Here's the drawing with two shaded views (mm, measured from the low corner). I have some questions. A direction names the side the tool comes from. Round coordinates to 2 decimals unless told otherwise and drop trailing zeros. Order: outer loops, then holes, each group sorted by start corner. A loop starts at its lowest first (then second) coordinate and runs counter-clockwise, first axis right, second up. Notation, with made-up numbers: (-15.5, 62.25) -> (23.5, 62.25) arc R26 ccw to (23.5, 86.25) -> close; hole circle Ø7 at (1, 39.5). An arc over 180 degrees is marked (long way). Use a Markdown table: item, result. Add a question column.
Q1. I need wall thicknesses on line 1 along Y through (x, z) = (3.1, 3.85); line 2 along Y through (x, z) = (0.5, 4); line 3 along X through (y, z) = (12.15, 4.05). Which ranges of each line are inside material? Lowest first, please. Write a range as [from, to].
Q2. For the marked faces 1 and 2, which set-ups out of +Z, -Z, +X, -X, +Y, -Y let a thin tool reach every point of the face, with its end or its side?
Q3. We'd pull the mould along X, two halves only. Please class the marked faces 3, 4 and 5: +X half, -X half, draft (parallel to the pull), parting line (faces both ways), or undercut.
Q4. If we section it at A-A on x = 3.1: List the corners of the cut face in (y, z) for me.
Q5. If we section it at C-C on y = 9.25: List the corners of the cut face in (x, z) for me, plus the area to 3 significant figures.
Q6. If we section it at D-D on x = 4.75: List the corners of the cut face in (y, z) for me.
Q7. If we section it at B-B on z = 3.1: List the corners of the cut face in (x, y) for me.
Q8. I'm going to push flat-ended pins straight in: pin 1 Ø1 at (x, z) = (2.5, 5.5) entering from -Y; pin 2 Ø2 at (x, y) = (3, 4.5) entering from -Z. Where does each tip first touch, or does it pass through?
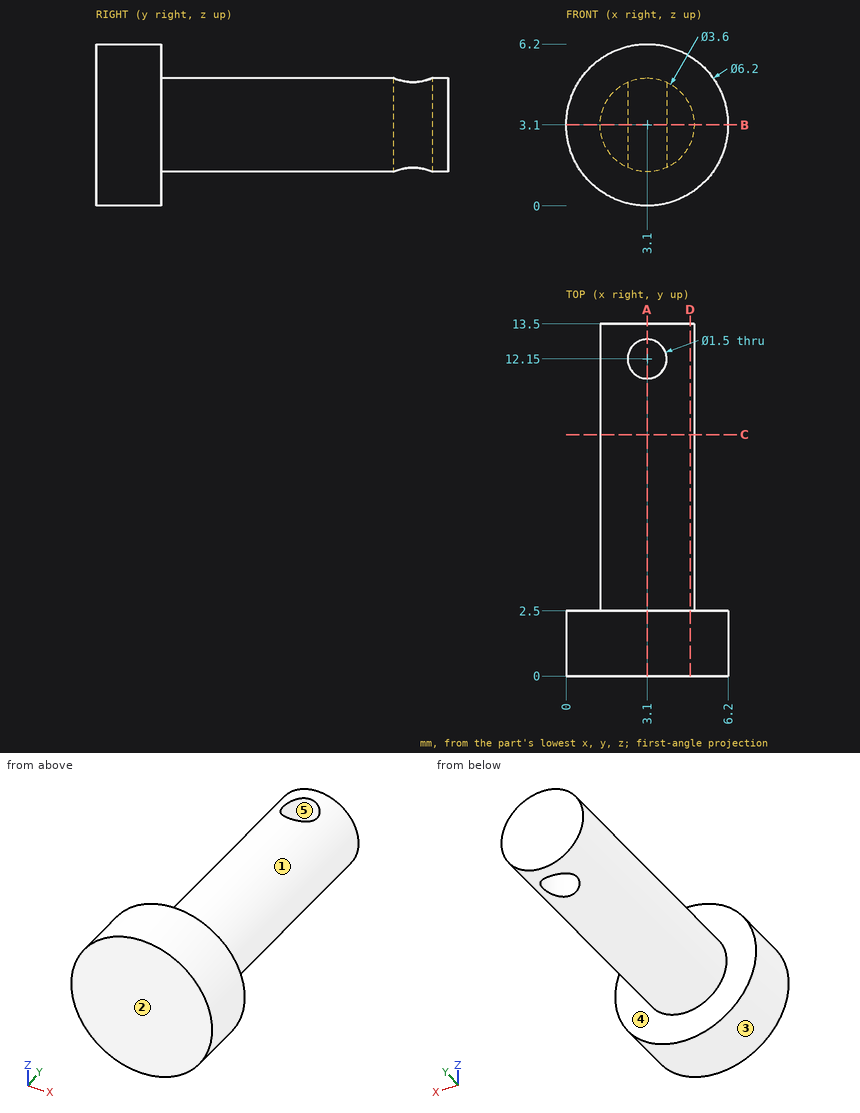
Answer below:
| question | item | result |
|---|---|---|
| 1 | line 1 | [0, 11.4], [12.9, 13.5] |
| 1 | line 2 | [0, 2.5] |
| 1 | line 3 | [1.57, 2.35], [3.85, 4.63] |
| 2 | face 1 | +Y |
| 2 | face 2 | +Z, -Z, +X, -X, -Y |
| 3 | face 3 | parting line |
| 3 | face 4 | draft |
| 3 | face 5 | undercut |
| 4 | outline | (0, 0) -> (2.5, 0) -> (2.5, 1.3) -> (11.4, 1.3) -> (11.4, 4.9) -> (2.5, 4.9) -> (2.5, 6.2) -> (0, 6.2) -> close; (12.9, 1.3) -> (13.5, 1.3) -> (13.5, 4.9) -> (12.9, 4.9) -> close |
| 5 | outline | circle Ø3.6 at (3.1, 3.1) |
| 5 | area | 10.2 mm² |
| 6 | outline | (0, 0.48) -> (2.5, 0.48) -> (2.5, 2.38) -> (13.5, 2.38) -> (13.5, 3.82) -> (2.5, 3.82) -> (2.5, 5.72) -> (0, 5.72) -> close |
| 7 | outline | (0, 0) -> (6.2, 0) -> (6.2, 2.5) -> (4.9, 2.5) -> (4.9, 13.5) -> (1.3, 13.5) -> (1.3, 2.5) -> (0, 2.5) -> close; hole circle Ø1.5 at (3.1, 12.15) |
| 8 | pin 1 | y = 0 |
| 8 | pin 2 | z = 1.3 |
